```python
from build123d import *

# Parameters (mm, degrees)
F0_R     = 11
F0_R_2   = 7.9
F1_DEPTH = 7
F2_R     = 2


with BuildPart() as f1:
    # F0 (on Top) → F1 (new body)
    with BuildSketch(Plane.XY):
        with BuildLine():
            ThreePointArc((-9.4396769012, 29.65), (-5.6554937849, 20.2702904388), (-8.9990265356, 10.7246222037))
            ThreePointArc((-8.9990265356, 10.7246222037), (0, -14), (8.9990265356, 10.7246222037))
            ThreePointArc((8.9990265356, 10.7246222037), (5.6554937849, 20.2702904388), (9.4396769012, 29.65))
            ThreePointArc((9.4396769012, 29.65), (0, 46), (-9.4396769012, 29.65))
        make_face()
        Circle(F0_R, mode=Mode.SUBTRACT)
        with Locations((0, 35.1)):
            Circle(F0_R_2, mode=Mode.SUBTRACT)
    extrude(amount=F1_DEPTH)

    # F2 (call 1 of 2: OpenCascade refuses the feature's edges together)
    f2_edges = [f1.edges().sort_by_distance(p)[0] for p in [
        (-5.655494, 20.27029, 7),
        (0, 46, 7),
        (5.655494, 20.27029, 7),
        (0, -14, 7),
    ]]
    fillet(f2_edges, radius=F2_R)

    # F2#2 (call 2 of 2)
    f2_2_edges = [f1.edges().sort_by_distance(p)[0] for p in [
        (0, -14, 0),
        (5.655494, 20.27029, 0),
        (0, 46, 0),
        (-5.655494, 20.27029, 0),
    ]]
    fillet(f2_2_edges, radius=F2_R)


solid = f1.part
```
Part model, mm, in its own coordinate system. Coordinates: 2 decimals unless noted, no trailing zeros. Order: outer loops, then holes, each group sorted by start corner. A loop starts at its lowest first (then second) coordinate and runs counter-clockwise, first axis right, second up. Notation, with made-up numbers: (9, 88) -> (49, 88) arc R27 ccw to (49, 108) -> close; hole circle Ø9 at (-32, 64). An arc over 180 degrees is marked (long way). Put each result on its own line as item: value. Start each with the question number.
(1) Band-saw the part on B-B (z = 3.75). Give the cut face in (x, y), then the cut area to 3 significant figures.
(2) Probe line 1 along Y through (x, z) = (-3.75, 1.5); line 2 along Y through (x, z) = (7.25, 2.5); line 3 along Y through (x, z) = (9.5, 2). List the from-to ranges inside material, lowest first. Write a range as [from, to].
(3) Band-saw the part on C-C (z = 1.25). Count the separate pieces of the cut face and the enclosed holes in it, then the cut area to 3 significant figures.
(4) Band-saw the part on A-A (x = 0). Give the cut face in (y, z), then the cut area to 3 significant figures.
(5) Mould opens along X. For faces 1 (the face through (0, 46, 3)), 2 (the face through (-1.713, 27.388, 3.451)), 3 (the face through (5.653, 20.126, 3.479)), 4 (the face through (-2.38, -10.74, 3.45)) say: pulls with the +X half, pulls with the -X half, needs draft (parallel to the pull), parting line crosses it, or undercut.
(6) Pin check, flat tips, straight feed: pin 1 Ø2 at (y, z) = (1, 0.5) entering from -X; pin 2 Ø14 at (x, y) = (0, 35.1) entering from -Z; pin 3 Ø1.5 at (y, z) = (8, 4) entering from -X; pin 4 Ø4 at (y, z) = (18.5, 1) entering from -X. Stop position of each tip, or through.
Determined:
1. outline: (-9.44, 29.65) arc R14.35 cw to (-9, 10.72) arc R14 ccw (long way) to (9, 10.72) arc R14.35 cw to (9.44, 29.65) arc R10.9 ccw (long way) to start; hole circle Ø22 at (0, 0); hole circle Ø15.8 at (0, 35.1)
1. area: 556 mm²
2. line 1: y = [-13.42, -10.34], [10.34, 28.15], [42.05, 45.27]
2. line 2: y = [-11.98, -8.27], [8.27, 13.35], [26.52, 31.96], [38.24, 43.24]
2. line 3: y = [-10.28, -5.55], [5.55, 10.28], [29.76, 40.44]
3. separate pieces: 1
3. enclosed holes: 2
3. area: 533 mm²
4. outline: (-14, 2) arc R2 ccw to (-12, 0) -> (-11, 0) -> (-11, 7) -> (-12, 7) arc R2 ccw to (-14, 5) -> close; (11, 0) -> (27.2, 0) -> (27.2, 7) -> (11, 7) -> close; (43, 0) -> (44, 0) arc R2 ccw to (46, 2) -> (46, 5) arc R2 ccw to (44, 7) -> (43, 7) -> close
4. area: 152 mm²
5. face 1: parting line crosses it
5. face 2: undercut
5. face 3: pulls with the +X half
5. face 4: undercut
6. pin 1: stops at x = -13.91
6. pin 2: passes through
6. pin 3: stops at x = -11.98
6. pin 4: stops at x = -6.02
